from build123d import *

# Parameters (mm, degrees)
SKETCH1_R           = 0.75
BOSS_EXTRUDE1_DEPTH = 1.4
FILLET1_R           = 0.5


with BuildPart() as part:
    # Sketch1 → Boss-Extrude1 (new body)
    with BuildSketch(Plane.XY):
        Polygon((-2.25, 2), (-2.25, -2), (2.75, -2), (5.25, -0.5), (5.25, 2), align=None)
        Circle(SKETCH1_R, mode=Mode.SUBTRACT)
    extrude(amount=BOSS_EXTRUDE1_DEPTH)

    # Fillet1
    fillet1_edges = [part.edges().sort_by_distance(p)[0] for p in [
        (5.25, 0.75, 0),
        (4, -1.25, 0),
        (0.25, -2, 0),
        (-2.25, 0, 0),
        (1.5, 2, 0),
    ]]
    fillet(fillet1_edges, radius=FILLET1_R)


solid = part.part
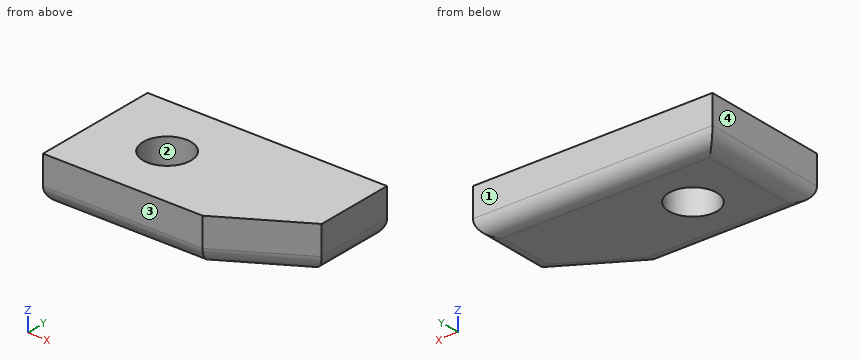
Verification items for the finished model (mm, model axes). Face numbers are marked on the shaded views. Give positions to 0.01 mm unless a question says otherwise; leave off trailing zeros. Write each loop counter-clockwise with the first axis right and the second up, starting at its lowest first coordinate (ties: lowest second). Pieces come first, ordered by that corner, then holes. Notation, with made-up numbers: M -30,41 L 11,41 A35 ccw 11,73 Z; hole C -20,23 d2. An arc over 180 degrees is marked long. Put each result on its own line as item: value. Start each with the question number.
1. Section check A-A (y = 0). Record the cut outline in (x, z), and give its area (3 significant figures).
2. Section check D-D (x = 2). Record the cut outline in (y, z), and give its area (3 significant figures).
3. Draft check along Y on the marked faces 1, 2, 3 and 4. Enter one of: +Y half, -Y half, draft (parallel to the pull), parting line (faces both ways), or undercut.
4. Section check C-C (z = 0.75). Record the cut outline in (x, y).
5. Section check B-B (x = 0). Record the cut outline in (y, z), and give its area (3 significant figures).
6. Scan lines: line 1 along Y through (x, z) = (0, 0.8); line 2 along X through (y, z) = (0.45, 1.15); line 3 along X through (y, z) = (0.55, 0.35). Record each from-to range of solid material in increasing order. Write a range as [from, to].
Answer list:
1. outline: M -2.25,0.5 A0.5 ccw -1.75,0 L -0.75,0 L -0.75,1.4 L -2.25,1.4 Z; M 0.75,0 L 4.75,0 A0.5 ccw 5.25,0.5 L 5.25,1.4 L 0.75,1.4 Z
1. area: 8.29 mm2
2. outline: M -2,0.5 A0.5 ccw -1.5,0 L 1.5,0 A0.5 ccw 2,0.5 L 2,1.4 L -2,1.4 Z
2. area: 5.49 mm2
3. face 1: +Y half
3. face 2: undercut
3. face 3: -Y half
3. face 4: draft
4. outline: M -2.25,-2 L 2.75,-2 L 5.25,-0.5 L 5.25,2 L -2.25,2 Z; hole C 0,0 d1.5
5. outline: M -2,0.5 A0.5 ccw -1.5,0 L -0.75,0 L -0.75,1.4 L -2,1.4 Z; M 0.75,0 L 1.5,0 A0.5 ccw 2,0.5 L 2,1.4 L 0.75,1.4 Z
5. area: 3.39 mm2
6. line 1: [-2, -0.75], [0.75, 2]
6. line 2: [-2.25, -0.6], [0.6, 5.25]
6. line 3: [-2.23, -0.51], [0.51, 5.23]
